The listing builds one solid part. Answer for the finished solid, in the listing's coordinates (mm). A direction names the side the tool comes from. Coordinates: 2 decimals unless noted, no trailing zeros. Order: outer loops, then holes, each group sorted by start corner. A loop starts at its lowest first (then second) coordinate and runs counter-clockwise, first axis right, second up.
from build123d import *

# Parameters (mm, degrees)
SKETCH1_W               = 390
SKETCH1_H               = 390
SKETCH1_W_2             = 350
SKETCH1_H_2             = 350
BOSS_EXTRUDE1_DEPTH     = 20
SKETCH2_W               = 20
SKETCH2_H               = 20
BOSS_EXTRUDE2_DEPTH     = 100
SKETCH4_W               = 390
SKETCH4_H               = 20
BOSS_EXTRUDE3_DEPTH     = 20
CUT_EXTRUDE1_DEPTH      = 448.353327919
CUT_EXTRUDE1_DEPTH_BACK = 448.353327919
SKETCH5_W               = 350
SKETCH5_H               = 20


with BuildPart() as part:
    # Sketch1 → Boss-Extrude1 (new body)
    with BuildSketch(Plane(origin=(0, 0, 0), x_dir=(1, 0, 0), z_dir=(0, 1, 0))):
        Rectangle(SKETCH1_W, SKETCH1_H)
        Rectangle(SKETCH1_W_2, SKETCH1_H_2, mode=Mode.SUBTRACT)
    extrude(amount=BOSS_EXTRUDE1_DEPTH)

    # Sketch2 → Boss-Extrude2 (add)
    with BuildSketch(Plane.XZ):
        with Locations((-185, 185)):
            Rectangle(SKETCH2_W, SKETCH2_H)
        with Locations((185, 185)):
            Rectangle(SKETCH2_W, SKETCH2_H)
        with Locations((185, -185)):
            Rectangle(SKETCH2_W, SKETCH2_H)
        with Locations((-185, -185)):
            Rectangle(SKETCH2_W, SKETCH2_H)
    extrude(amount=BOSS_EXTRUDE2_DEPTH)

    # Sketch4 → Boss-Extrude3 (add)
    with BuildSketch(Plane(origin=(0, 20, 0), x_dir=(1, 0, 0), z_dir=(0, 1, 0))):
        with Locations((0, -185)):
            Rectangle(SKETCH4_W, SKETCH4_H)
        with Locations((0, 185)):
            Rectangle(SKETCH4_W, SKETCH4_H)
    extrude(amount=BOSS_EXTRUDE3_DEPTH)

    # Sketch5 → Cut-Extrude1 (cut, two sides: drawn at the far end of the back side and taken through both)
    with BuildSketch(Plane.XY.offset(195).offset(-CUT_EXTRUDE1_DEPTH_BACK)):
        with Locations((0, 10)):
            Rectangle(SKETCH5_W, SKETCH5_H)
    extrude(amount=CUT_EXTRUDE1_DEPTH + CUT_EXTRUDE1_DEPTH_BACK, mode=Mode.SUBTRACT)


solid = part.part
1) Section B-B (y = -73.5) is taken. Give the vertices of the cut face in (x, z), then the cut area to 3 significant figures.
2) A tool of negligible diameter and unlimited length cuts with its end or side. For faces 1 (the face through (-185, 20, -2)), 2 (the face through (185, 0, -2)), 3 (the face through (-185, -100, -185)), from which of +Z, -Z, +X, -X, +Y, -Y can it reach the whole face along a straight path? Write none if from no direction.
3) Determine the mould class of faces 4 (the face through (185, 20, -2)), 5 (the face through (-2, 20, -185)), 6 (the face through (-175, 9, 1)), 7 (the face through (195, 6, 1)) for opening direction X: released by +X, released by -X, zero draft, split by the parting line, or undercut.
4) Section A-A (x = -127) is taken. Give the vertices of the cut face in (y, z).
5) Section C-C (z = -31) is taken. Give the vertices of the cut face in (x, y), then the cut area to 3 significant figures.
6) Each of these flat-tipped pins is pushed along its axis until it touches: P1, Ø10, axis at x = 188, z = -38, coming from the -Y side; P2, Ø16, axis at x = -4.5, z = -188, coming from the -Y side; P3, Ø10, axis at x = -181.5, z = 59, coming from the +Y side. Where does it stop, or does it pass through?
7) Consider L1, parallel to X at y = 1, z = 123. Determine where the line is inside the solid, lowest interval first.
Filled sheet:
1. outline: (-195, -195) - (-175, -195) - (-175, -175) - (-195, -175) - close; (-195, 175) - (-175, 175) - (-175, 195) - (-195, 195) - close; (175, -195) - (195, -195) - (195, -175) - (175, -175) - close; (175, 175) - (195, 175) - (195, 195) - (175, 195) - close
1. area: 1,600 mm2
2. face 1: +X, -X, +Y
2. face 2: +X, -X, -Y
2. face 3: +Z, -Z, +X, -X, -Y
3. face 4: zero draft
3. face 5: undercut
3. face 6: undercut
3. face 7: released by +X
4. outline: (20, -195) - (40, -195) - (40, -175) - (20, -175) - close; (20, 175) - (40, 175) - (40, 195) - (20, 195) - close
5. outline: (-195, 0) - (-175, 0) - (-175, 20) - (-195, 20) - close; (175, 0) - (195, 0) - (195, 20) - (175, 20) - close
5. area: 800 mm2
6. P1: stops at y = 0
6. P2: stops at y = 20
6. P3: stops at y = 20
7. L1: x = -195 to -175, 175 to 195
